The listing builds one solid part. Answer for the finished solid, in the listing's coordinates (mm). Face numbers are marked on the shaded views. A direction names the side the tool comes from. Coordinates: 2 decimals unless noted, no trailing zeros. Order: outer loops, then holes, each group sorted by start corner. A loop starts at its lowest first (then second) coordinate and runs counter-clockwise, first axis right, second up. Notation, with made-up numbers: M 23,-21 L 66,-21 A20 ccw 66,-6 Z; hole C 82.25,21 d8. An arc over 180 degrees is marked long. One line per item, written item: value. Start each with the question number.
Q1. The part is cut by section A-A on x = 82.5. Give the vertices of the cut face in (y, z).
Q2. Each of these flat-tipped pins is pushed along its axis until it touches: pin 1 Ø8 at (x, z) = (35, -47.5) entering from -Y; pin 2 Ø3 at (x, z) = (159.5, 28.5) entering from +Y; pin 3 Ø5 at (x, z) = (89.5, -44.5) entering from -Y; pin 4 Ø11 at (y, z) = (16.5, -48) entering from -X. Where does it stop, or does it pass through?
Q3. The part is cut by section B-B on y = 10. Give the vertices of the cut face in (x, z).
Q4. Determine the mould class of the marked faces 6, 7 and 8 for opening direction Z: pulls with the +Z half, pulls with the -Z half, needs draft (parallel to the pull), parting line crosses it, or undercut.
Q5. The part is cut by section D-D on x = 29. Give the vertices of the cut face in (y, z), then the cut area to 3 significant figures.
Q6. The part is cut by section C-C on z = 29. Give the vertices of the cut face in (x, y), then the cut area to 3 significant figures.
Q7. Straight lines are drawn through the part: line 1 along X through (y, z) = (4, -46); line 2 along Z through (x, y) = (32, -56); line 3 along Z through (x, y) = (13, 5.5). For each, find the intervals that lie inside material, in ascending order. Write a range as [from, to].
Q8. For the marked faces 1, 2, 3, 4 and 5, determine the directions among +Z, -Z, +X, -X, +Y, -Y from which every point of the face is accessible in a straight line to the end or side of a thin tool.
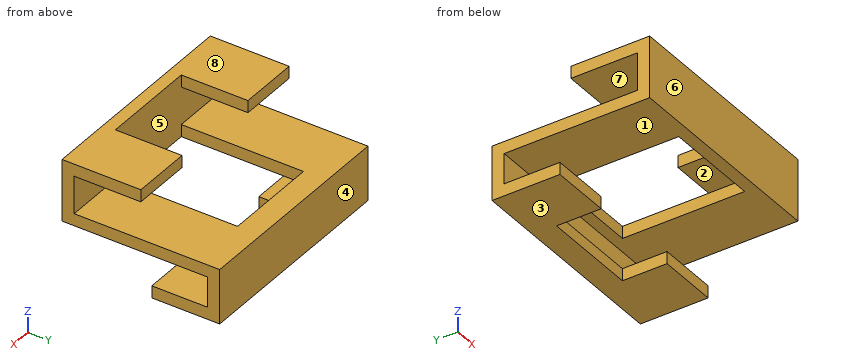
```python
from build123d import *

# Parameters (mm, degrees)
BOSS_EXTRUDE1_DEPTH     = 180
CUT_EXTRUDE1_DEPTH      = 202.244874193
CUT_EXTRUDE1_DEPTH_BACK = 202.244874193
SKETCH3_W               = 80
SKETCH3_H               = 100.784598353


with BuildPart() as part:
    # Sketch1 → Boss-Extrude1 (new body)
    with BuildSketch(Plane(origin=(0, 0, 0), x_dir=(0, 0, -1), z_dir=(1, 0, 0))):
        Polygon((41.824095604, 42.060925147), (41.824095604, -3.939074853), (51.824095604, -3.939074853), (51.824095604, 52.060925147), (6.824095604, 52.060925147), (6.824095604, -77.939074853), (16.824095604, -77.939074853), (16.824095604, 42.060925147), align=None)
        Polygon((6.824095604, -77.939074853), (6.824095604, -67.939074853), (-24.175904396, -67.939074853), (-24.175904396, -12.939074853), (-34.175904396, -12.939074853), (-34.175904396, -77.939074853), align=None)
    extrude(amount=BOSS_EXTRUDE1_DEPTH)

    # Sketch3 → Cut-Extrude1 (cut, two sides: drawn at the far end of the back side and taken through both)
    with BuildSketch(Plane.XY.offset(-6.824095604).offset(-CUT_EXTRUDE1_DEPTH_BACK)):
        with Locations((90, -17.546775677)):
            Rectangle(SKETCH3_W, SKETCH3_H)
    extrude(amount=CUT_EXTRUDE1_DEPTH + CUT_EXTRUDE1_DEPTH_BACK, mode=Mode.SUBTRACT)


solid = part.part
```
Output:
1. outline: M -77.94,-16.82 L -67.94,-16.82 L -67.94,34.18 L -77.94,34.18 Z; M 32.85,-51.82 L 52.06,-51.82 L 52.06,-6.82 L 32.85,-6.82 L 32.85,-16.82 L 42.06,-16.82 L 42.06,-41.82 L 32.85,-41.82 Z
2. pin 1: stops at y = -3.94
2. pin 2: stops at y = -12.94
2. pin 3: stops at y = 32.85
2. pin 4: stops at x = 0
3. outline: M 0,-51.82 L 50,-51.82 L 50,-41.82 L 0,-41.82 Z; M 0,-16.82 L 50,-16.82 L 50,-6.82 L 0,-6.82 Z; M 130,-51.82 L 180,-51.82 L 180,-41.82 L 130,-41.82 Z; M 130,-16.82 L 180,-16.82 L 180,-6.82 L 130,-6.82 Z
4. face 6: needs draft
4. face 7: undercut
4. face 8: pulls with the +Z half
5. outline: M -77.94,-16.82 L 42.06,-16.82 L 42.06,-41.82 L -3.94,-41.82 L -3.94,-51.82 L 52.06,-51.82 L 52.06,-6.82 L -67.94,-6.82 L -67.94,24.18 L -12.94,24.18 L -12.94,34.18 L -77.94,34.18 Z
5. area: 3,070 mm^2
6. outline: M 0,-77.94 L 180,-77.94 L 180,-12.94 L 130,-12.94 L 130,-67.94 L 50,-67.94 L 50,-12.94 L 0,-12.94 Z
6. area: 7,300 mm^2
7. line 1: x = [0, 50], [130, 180]
7. line 2: z = [-16.82, -6.82], [24.18, 34.18]
7. line 3: z = [-51.82, -41.82], [-16.82, -6.82]
8. face 1: +X, -X, -Y
8. face 2: +X, -X, +Y
8. face 3: -Z, +X, -X, +Y, -Y
8. face 4: +Z, -Z, +X, -X, +Y
8. face 5: none
